For this review, take the finished solid that the model builds, in its own axes (mm). Round coordinates to 2 decimals unless told otherwise and drop trailing zeros. Order: outer loops, then holes, each group sorted by start corner. A loop starts at its lowest first (then second) coordinate and runs counter-clockwise, first axis right, second up. Notation, with made-up numbers: M -28,-22 L 21,-22 A16 cw 21,-8 Z; hole C 44.5,-4.5 d1. An arc over 180 degrees is marked long. Answer in a Markdown table with one row per item. Add a question column.
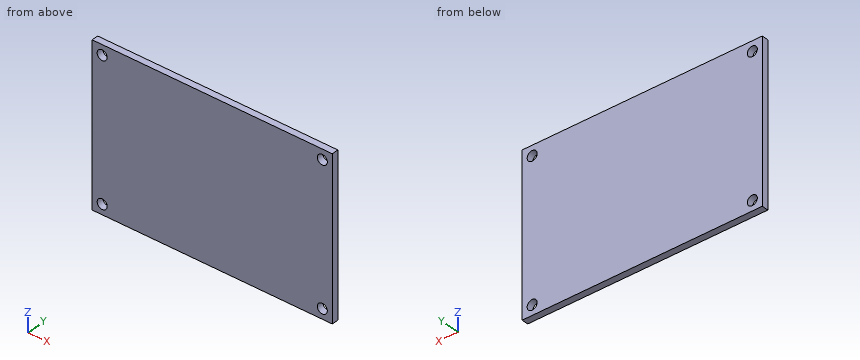
Autodesk Inventor part; units mm, degrees
ref_plane "YZ Plane" through (0, 0, 0) normal (1, 0, 0) x (0, 1, 0)
ref_plane "XZ Plane" through (0, 0, 0) normal (0, 1, 0) x (-1, 0, 0)
ref_plane "XY Plane" through (0, 0, 0) normal (0, 0, 1) x (1, 0, 0)
sketch "スケッチ1" plane through (0, 0, 0) normal (0, 1, 0) x (-1, 0, 0)
  line L0 (36, 24) -> (-36, 24)
  line L1 (-36, 24) -> (-36, -24)
  line L2 (-36, -24) -> (36, -24)
  line L3 (36, -24) -> (36, 24)
  line L4 (36, 24) -> (-36, -24) construction
  line L5 (-36, 24) -> (36, -24) construction
  circle A0 centre (33, 21) radius 1.5
  line L6 (50.4, 0) -> (-50.4, 0) construction
  circle A1 centre (33, -21) radius 1.5
  line L7 (0, -33.6) -> (0, 33.6) construction
  circle A2 centre (-33, 21) radius 1.5
  circle A3 centre (-33, -21) radius 1.5
  point P0 (0, 0)
  dimension "d0" = 48
  dimension "d1" = 72
  dimension "d2" = 3
  dimension "d3" = 3
  dimension "d4" = 42
extrude "押し出し1" add sketch "スケッチ1" along normal blind 2
properties part number "circuitboard"
1. Consider section A-A on x = 33. Write out the cut boundary in (y, z), plus the area to 3 significant figures.
2. Consider section B-B on z = -21. Write out the cut boundary in (x, y), plus the area to 3 significant figures.
3. To check wall thickness, follow probe 1 along Z at (x, y) = (33, 0.8). State the ranges of the line that lie inside material, in increasing order. Write a range as [from, to].
4. Clearance check with a flat-ended pin moving along its axis: pin 1 Ø2.5 at (x, z) = (33, 21) entering from +Y. State where the tip first meets the part, or that it passes through.
Solved:
| question | item | result |
|---|---|---|
| 1 | outline | M 0,-24 L 2,-24 L 2,-22.5 L 0,-22.5 Z; M 0,-19.5 L 2,-19.5 L 2,19.5 L 0,19.5 Z; M 0,22.5 L 2,22.5 L 2,24 L 0,24 Z |
| 1 | area | 84.0 mm^2 |
| 2 | outline | M -36,0 L -34.5,0 L -34.5,2 L -36,2 Z; M -31.5,0 L 31.5,0 L 31.5,2 L -31.5,2 Z; M 34.5,0 L 36,0 L 36,2 L 34.5,2 Z |
| 2 | area | 132 mm^2 |
| 3 | probe 1 | z = [-24, -22.5], [-19.5, 19.5], [22.5, 24] |
| 4 | pin 1 | passes through |
